Geometry: final body of the model. Coordinates: model frame, mm. Face numbers are marked on the shaded views. A direction names the side the tool comes from. Give positions to 0.01 mm unless a question says otherwise; leave off trailing zeros. Write each loop counter-clockwise with the first axis right and the second up, starting at its lowest first coordinate (ties: lowest second). Pieces come first, ordered by that corner, then holes. Notation, with made-up numbers: M 74.25,12 L 110.25,12 A22 ccw 110.25,40 Z; hole C -31,-40 d8. An arc over 180 degrees is marked long. Use one line per item in the form item = value. Start each with the question number.
Item 1: Section query C-C on y = 6.5. Return loops of the section in (x, z).
Item 2: Material intervals for line 1 along X through (y, z) = (2.25, 0); line 2 along X through (y, z) = (7, 0); line 3 along Y through (x, z) = (-7, -18.5), sorted ascending. Write a range as from..to.
Item 3: Section query A-A on x = 0. Return loops of the section in (y, z), then the cut area to 3 significant figures.
Item 4: Pull-direction query (X, two-part tool) for the marked faces 1, 2 and 3; classes: released by +X, released by -X, zero draft, split by the parting line, or undercut.
Item 5: Section query B-B on z = 0. Return loops of the section in (x, y), then the cut area to 3 significant figures.
Item 6: Contact query for flat-ended pins moving along their axis: P1, Ø2, axis at x = -11, z = -24, coming from the -Y side; P2, Ø21, axis at x = 5, z = -6, coming from the +Y side; P3, Ø1.5, axis at y = 8.5, z = 7, coming from the -X side; P4, Ø1.5, axis at x = 20, y = 8.5, coming from the +Z side. Output: stop coordinate, or through.
Item 7: Section query D-D on x = 18.5. Return loops of the section in (y, z), then the cut area to 3 significant figures.
Item 8: Access query for the marked faces 4 and 5. Directions: +Z, -Z, +X, -X, +Y, -Y. A direction counts if a zero-diameter tool reaches every point of the face in a straight line with its end or side. Return the directions, or none.
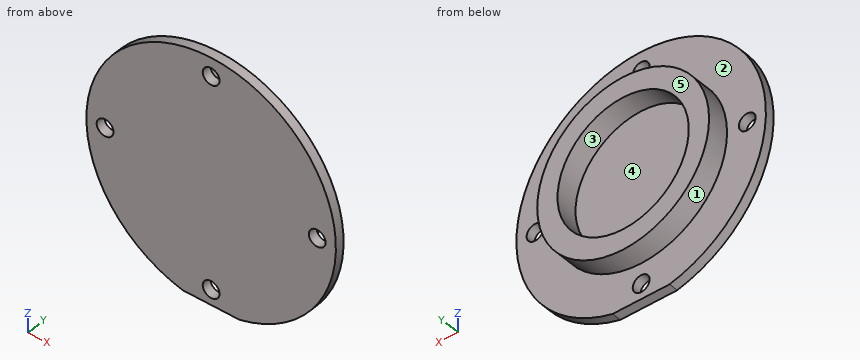
from build123d import *

# Parameters (mm, degrees)
SKETCH1_R           = 2.7
BOSS_EXTRUDE1_DEPTH = 3
SKETCH2_R           = 27.55
SKETCH2_R_2         = 21.05
BOSS_EXTRUDE2_DEPTH = 7


with BuildPart() as part:
    # Sketch1 → Boss-Extrude1 (new body)
    with BuildSketch(Plane(origin=(0, 0, 0), x_dir=(1, 0, 0), z_dir=(0, 1, 0))):
        with BuildLine():
            Line((-9.11971668, 38.946511624), (9.11971668, 38.946511624))
            ThreePointArc((9.11971668, 38.946511624), (0, -40), (-9.11971668, 38.946511624))
        make_face()
        with Locations(Location((0, 34.007379053, 0), (0, 0, 270))):
            Circle(SKETCH1_R, mode=Mode.SUBTRACT)
        with Locations(Location((34.007379053, 0, 0), (0, 0, 270))):
            Circle(SKETCH1_R, mode=Mode.SUBTRACT)
        with Locations(Location((-34.007379053, 0, 0), (0, 0, 270))):
            Circle(SKETCH1_R, mode=Mode.SUBTRACT)
        with Locations(Location((0, -34.007379053, 0), (0, 0, 270))):
            Circle(SKETCH1_R, mode=Mode.SUBTRACT)
    extrude(amount=BOSS_EXTRUDE1_DEPTH)

    # Sketch2 → Boss-Extrude2 (add)
    with BuildSketch(Plane(origin=(0, 3, 0), x_dir=(1, 0, 0), z_dir=(0, 1, 0))):
        with Locations(Location((0, 0, 0), (0, 0, 270))):
            Circle(SKETCH2_R)
        with Locations(Location((0, 0, 0), (0, 0, 270))):
            Circle(SKETCH2_R_2, mode=Mode.SUBTRACT)
    extrude(amount=BOSS_EXTRUDE2_DEPTH)


solid = part.part
Answer sheet:
q1.outline = C 0,0 d55.1; hole C 0,0 d42.1
q2.line_1 = -40..-36.71, -31.31..31.31, 36.71..40
q2.line_2 = -27.55..-21.05, 21.05..27.55
q2.line_3 = 0..3
q3.outline = M 0,-38.95 L 3,-38.95 L 3,-36.71 L 0,-36.71 Z; M 0,-31.31 L 3,-31.31 L 3,-27.55 L 10,-27.55 L 10,-21.05 L 3,-21.05 L 3,21.05 L 10,21.05 L 10,27.55 L 3,27.55 L 3,31.31 L 0,31.31 Z; M 0,36.71 L 3,36.71 L 3,40 L 0,40 Z
q3.area = 295 mm2
q4.face_1 = split by the parting line
q4.face_2 = zero draft
q4.face_3 = undercut
q5.outline = M -40,0 L -36.71,0 L -36.71,3 L -40,3 Z; M -31.31,0 L 31.31,0 L 31.31,3 L 27.55,3 L 27.55,10 L 21.05,10 L 21.05,3 L -21.05,3 L -21.05,10 L -27.55,10 L -27.55,3 L -31.31,3 Z; M 36.71,0 L 40,0 L 40,3 L 36.71,3 Z
q5.area = 299 mm2
q6.P1 = 0
q6.P2 = 3
q6.P3 = -26.83
q6.P4 = 19.71
q7.outline = M 0,-35.46 L 3,-35.46 L 3,-20.41 L 10,-20.41 L 10,-10.04 L 3,-10.04 L 3,10.04 L 10,10.04 L 10,20.41 L 3,20.41 L 3,35.46 L 0,35.46 Z
q7.area = 358 mm2
q8.face_4 = +Y
q8.face_5 = +Z, -Z, +X, -X, +Y
